The model under review builds one solid part; all positions refer to its coordinate system, in mm. A direction names the side the tool comes from. Coordinates: 2 decimals unless noted, no trailing zeros. Order: outer loops, then holes, each group sorted by start corner. A loop starts at its lowest first (then second) coordinate and runs counter-clockwise, first axis right, second up.
```python
from build123d import *

# Parameters (mm, degrees)
F1_DEPTH = 4.572
F2_R     = 1.4097
F3_DEPTH = 6.0325
F4_W     = 3.81
F4_H     = 3.937
F5_DEPTH = 1.6256
F7_DEPTH = 1.651
F9_DEPTH = 2.413


with BuildPart() as f1:
    # F0 (on Top) → F1 (new body, symmetric)
    with BuildSketch(Plane.XY):
        with BuildLine():
            Line((-3.174979, -4.71263), (-1.1303, -4.71263))
            Line((-1.1303, -4.71263), (1.1303, -4.71263))
            Line((1.1303, -4.71263), (3.174979, -4.71263))
            ThreePointArc((3.174979, -4.71263), (2.611007, -2.917836), (1.1303, -1.757295))
            Line((1.1303, -1.757295), (1.1303, 3.278927))
            ThreePointArc((1.1303, 3.278927), (0, 6.71737), (-1.1303, 3.278927))
            Line((-1.1303, 3.278927), (-1.1303, -1.757295))
            ThreePointArc((-1.1303, -1.757295), (-2.611007, -2.917836), (-3.174979, -4.71263))
        make_face()
    extrude(amount=F1_DEPTH, both=True)

    # F2 (on Top) → F3 (join, symmetric)
    with BuildSketch(Plane.XY):
        with Locations((0, -4.71263)):
            Circle(F2_R)
    extrude(amount=F3_DEPTH, both=True)

    # F4 (on Top) → F5 (join, symmetric)
    with BuildSketch(Plane.XY):
        with Locations((0, -6.68113)):
            Rectangle(F4_W, F4_H)
    extrude(amount=F5_DEPTH, both=True)

    # F6 (on Top) → F7 (join, symmetric)
    with BuildSketch(Plane.XY):
        Polygon((3.3782, -8.64963), (-3.3782, -8.64963), (-2.701088, -12.89143), (2.658312, -12.89143), align=None)
    extrude(amount=F7_DEPTH, both=True)

    # F8 (on face) → F9 (join)
    with BuildSketch(Plane.XY.offset(1.651)):
        Polygon((1.143, -12.89143), (-1.143, -12.89143), (-0.950346, -15.93943), (0.954654, -15.93943), align=None)
    extrude(amount=-F9_DEPTH)


solid = f1.part
```
(1) We need section D-D, the plane z = 5.5. Write out the cut boundary in (x, y), and give its area (3 significant figures).
A:
outline: circle Ø2.82 at (0, -4.71)
area: 6.24 mm2
(2) Draft analysis for pull direction Y (two halves, no side actions). For faces 5 (the face through (0, -5, -6.032)), 6 (the face through (-0.306, -6.089, -4.288)), 7 (the face through (1.905, -7, 0)), state which applies: released by +Y, released by -Y, zero draft, split by the parting line, or undercut.
A:
face 5: zero draft
face 6: split by the parting line
face 7: undercut
(3) We need section B-B, the plane z = -4.25. Write out the cut boundary in (x, y) (3 decimals).
A:
outline: (-3.175, -4.713) - (-1.41, -4.713) arc R1.41 ccw to (1.41, -4.713) - (3.175, -4.713) arc R3.175 ccw to (1.13, -1.757) - (1.13, 3.279) arc R1.905 ccw (long way) to (-1.13, 3.279) - (-1.13, -1.757) arc R3.175 ccw to start
(4) Machinability: for faces 1 (the face through (0, -11, 1.651)), 2 (the face through (-1.905, -7, 0)), 3 (the face through (1.13, 1, 0)), 4 (the face through (2.3, -4.713, 0.1)), which of the approach directions +Z, -Z, +X, -X, +Y, -Y give a long, thin tool a straight path to every point of the face, cutting with its end or side? Answer none if there is none.
A:
face 1: +Z, +X, -X, -Y
face 2: +Z, -Z, -X
face 3: +Z, -Z, +X
face 4: +X
(5) For pin 1 Ø1 at (x, z) = (2, 0.5) entering from -Y; pin 2 Ø0.5 at (x, z) = (-2, 2) entering from -Y; pin 3 Ø3 at (x, y) = (-1, -6.5) entering from -Z; pin 4 Ø0.7 at (x, y) = (0, -14.5) entering from -Z, all flat-tipped, find the tip position at first contact; note any pin that passes through.
A:
pin 1: stops at y = -12.89
pin 2: stops at y = -4.71
pin 3: stops at z = -6.03
pin 4: stops at z = -0.76
(6) Wall thickness on probe 1 along Z at (x, y) = (-1, -7.75); probe 2 along Z at (x, y) = (1.5, -3): over which ranges is each line inside the solid? List them lowest first.
A:
probe 1: z = -1.63 to 1.63
probe 2: z = -4.57 to 4.57
(7) We need section C-C, the plane y = 2. Write out the cut boundary in (x, z).
A:
outline: (-1.13, -4.57) - (1.13, -4.57) - (1.13, 4.57) - (-1.13, 4.57) - close
